Geometry: final body of the model. Coordinates: model frame, mm. A direction names the side the tool comes from. Give positions to 0.01 mm unless a question says otherwise; leave off trailing zeros. Loops run counter-clockwise (first coordinate to the right, second up) from the corner with the lowest first, then second, coordinate; pieces in that order, holes last. Notation, with made-up numbers: M 51.25,26 L 106.25,26 A11 cw 106.25,33 Z; hole C -19.75,53.5 d1. An arc over 180 degrees is marked long. Put each result on its own line as item: value.
```python
from build123d import *

# Parameters (mm, degrees)
ESBO_O1_W                = 30
ESBO_O1_H                = 30
RESSALTO_EXTRUS_O1_DEPTH = 28.5
ESBO_O2_R                = 1.6
CORTE_EXTRUS_O1_DEPTH    = 5
ESBO_O3_R                = 2.25
RESSALTO_EXTRUS_O2_DEPTH = 3
ESBO_O4_W                = 15.5
ESBO_O4_H                = 20
RESSALTO_EXTRUS_O3_DEPTH = 12
ESBO_O5_R                = 2.25
RESSALTO_EXTRUS_O4_DEPTH = 5
RESSALTO_EXTRUS_O4_TAPER = 22
ESBO_O6_W                = 30
ESBO_O6_H                = 30
ESBO_O6_W_2              = 29.5
ESBO_O6_H_2              = 29.5
ESBO_O6_R                = 14.4
CORTE_EXTRUS_O2_DEPTH    = 10.5
RESSALTO_EXTRUS_O5_DEPTH = 6
ESBO_O10_R               = 5
RESSALTO_EXTRUS_O6_DEPTH = 5.5


with BuildPart() as part:
    # Esboço1 → Ressalto-extrusão1 (new body)
    with BuildSketch(Plane.XY):
        Rectangle(ESBO_O1_W, ESBO_O1_H)
    extrude(amount=RESSALTO_EXTRUS_O1_DEPTH)

    # Esboço2 → Corte-extrusão1 (cut)
    with BuildSketch(Plane(origin=(0, 0, 0), x_dir=(-1, 0, 0), z_dir=(0, 0, -1))):
        with Locations((4.5, 5)):
            Circle(ESBO_O2_R)
        with Locations((-4.5, 5)):
            Circle(ESBO_O2_R)
        with Locations((0, -4.8)):
            Circle(ESBO_O2_R)
    extrude(amount=-CORTE_EXTRUS_O1_DEPTH, mode=Mode.SUBTRACT)

    # Esboço3 → Ressalto-extrusão2 (add)
    with BuildSketch(Plane.XZ.offset(15)):
        with Locations((-9, 5.5)):
            Circle(ESBO_O3_R)
        with Locations((9, 5.5)):
            Circle(ESBO_O3_R)
    extrude(amount=RESSALTO_EXTRUS_O2_DEPTH)

    # Esboço4 → Ressalto-extrusão3 (add)
    with BuildSketch(Plane.XZ.offset(18)):
        with Locations((-9, 12)):
            Rectangle(ESBO_O4_W, ESBO_O4_H)
        with Locations((9, 12)):
            Rectangle(ESBO_O4_W, ESBO_O4_H)
    extrude(amount=RESSALTO_EXTRUS_O3_DEPTH)

    # Esboço5 → Ressalto-extrusão4 (add)
    with BuildSketch(Plane.XZ.offset(30)):
        with Locations((9, 5.5)):
            Circle(ESBO_O5_R)
        with Locations((-9, 5.5)):
            Circle(ESBO_O5_R)
    extrude(amount=RESSALTO_EXTRUS_O4_DEPTH, taper=RESSALTO_EXTRUS_O4_TAPER)

    # Esboço6 → Corte-extrusão2 (cut)
    with BuildSketch(Plane.XY.offset(28.5)):
        Rectangle(ESBO_O6_W, ESBO_O6_H)
        Rectangle(ESBO_O6_W_2, ESBO_O6_H_2, mode=Mode.SUBTRACT)
        Circle(ESBO_O6_R)
        with BuildLine():
            ThreePointArc((-7.846216259, 2.549390204), (-8.188505751, 1.005422083), (-8.229903415, -0.575490908))
            Line((-8.229903415, -0.575490908), (-13.866140299, -0.969614985))
            ThreePointArc((-13.866140299, -0.969614985), (-12.157213929, -6.738853721), (-8.170215007, -11.245336222))
            Line((-8.170215007, -11.245336222), (-4.849228331, -6.674390204))
            ThreePointArc((-4.849228331, -6.674390204), (-3.486600659, -7.477039243), (-1.995855639, -8.004939742))
            Line((-1.995855639, -8.004939742), (-3.362714349, -13.487110595))
            ThreePointArc((-3.362714349, -13.487110595), (2.652245036, -13.64461785), (8.170215007, -11.245336222))
            Line((8.170215007, -11.245336222), (4.849228331, -6.674390204))
            ThreePointArc((4.849228331, -6.674390204), (6.033668038, -5.626486471), (6.996396793, -4.37183393))
            Line((6.996396793, -4.37183393), (11.787868537, -7.365877773))
            ThreePointArc((11.787868537, -7.365877773), (13.796391508, -1.693983873), (13.219685577, 4.295336222))
            Line((13.219685577, 4.295336222), (7.846216259, 2.549390204))
            ThreePointArc((7.846216259, 2.549390204), (7.215612584, 3.999679367), (6.319866656, 5.30299778))
            Line((6.319866656, 5.30299778), (10.648017759, 8.934747775))
            ThreePointArc((10.648017759, 8.934747775), (5.874393838, 12.59767824), (0, 13.9))
            Line((0, 13.9), (0, 8.25))
            ThreePointArc((0, 8.25), (-1.574174212, 8.098424263), (-3.090504396, 7.6492668))
            Line((-3.090504396, 7.6492668), (-5.207031648, 12.887855578))
            ThreePointArc((-5.207031648, 12.887855578), (-10.165816453, 9.479777205), (-13.219685577, 4.295336222))
            Line((-13.219685577, 4.295336222), (-7.846216259, 2.549390204))
        make_face(mode=Mode.SUBTRACT)
    extrude(amount=-CORTE_EXTRUS_O2_DEPTH, mode=Mode.SUBTRACT)

    # Esboço9 → Ressalto-extrusão5 (add)
    with BuildSketch(Plane(origin=(0, 15, 0), x_dir=(1, 0, 0), z_dir=(0, 1, 0))):
        Polygon((14.773502692, -5.5), (11.886751346, -0.5), (6.113248654, -0.5), (3.226497308, -5.5), (6.113248654, -10.5), (11.886751346, -10.5), align=None)
        Polygon((-3.226497308, -5.5), (-6.113248654, -0.5), (-11.886751346, -0.5), (-14.773502692, -5.5), (-11.886751346, -10.5), (-6.113248654, -10.5), align=None)
    extrude(amount=RESSALTO_EXTRUS_O5_DEPTH)

    # Esboço10 → Ressalto-extrusão6 (add)
    with BuildSketch(Plane(origin=(0, 21, 0), x_dir=(1, 0, 0), z_dir=(0, 1, 0))):
        with Locations((-9, -5.5)):
            Circle(ESBO_O10_R)
        with Locations((9, -5.5)):
            Circle(ESBO_O10_R)
    extrude(amount=RESSALTO_EXTRUS_O6_DEPTH)


solid = part.part
```
Item 1: Line query: probe 1 along Y at (x, z) = (0, 3.1); probe 2 along Y at (x, z) = (-2, 6.25); probe 3 along X at (y, z) = (12, 21.5). Output: solid intervals per line, ascending. Write a range as [from, to].
Output values:
probe 1: [-15, -6.4], [-3.2, 15]
probe 2: [-30, -18], [-15, 15]
probe 3: [-14.75, -7.96], [-7.01, -4.85], [0, 7.01], [7.96, 14.75]
Item 2: Section C-C on z = 14.25. Output: boundary loops of the cut face in (x, y), then the cut area to 3 significant figures.
Output values:
outline: M -16.75,-30 L -1.25,-30 L -1.25,-18 L -16.75,-18 Z; M -15,-15 L 15,-15 L 15,15 L -15,15 Z; M 1.25,-30 L 16.75,-30 L 16.75,-18 L 1.25,-18 Z
area: 1,270 mm²
Item 3: Mould query, pull axis Y, two halves, no side actions, for faces 5 (the flat face through (13.31, 17.958, 8.035)), 6 (the flat face through (0, -5, 5)), 7 (the flat face through (6, 21, 10)). Classes: pulls with the +Y half, pulls with the -Y half, needs draft (parallel to the pull), parting line crosses it, or undercut.
Output values:
face 5: needs draft
face 6: undercut
face 7: pulls with the +Y half
Item 4: Section B-B on z = 24.5. Output: boundary loops of the cut face in (x, y), then the cut area to 3 significant figures.
Output values:
outline: M -14.75,-14.75 L 14.75,-14.75 L 14.75,14.75 L -14.75,14.75 Z; M -13.87,-0.97 A13.9 ccw -8.17,-11.25 L -4.85,-6.67 A8.25 ccw -2,-8 L -3.36,-13.49 A13.9 ccw 8.17,-11.25 L 4.85,-6.67 A8.25 ccw 7,-4.37 L 11.79,-7.37 A13.9 ccw 13.22,4.3 L 7.85,2.55 A8.25 ccw 6.32,5.3 L 10.65,8.93 A13.9 ccw 0,13.9 L 0,8.25 A8.25 ccw -3.09,7.65 L -5.21,12.89 A13.9 ccw -13.22,4.3 L -7.85,2.55 A8.25 ccw -8.23,-0.58 Z; hole C 0,0 d28.8
area: 706 mm²
Item 5: Set-up query: faces 1 (the cylindrical face through (-4.15, 3.44, 2.46)), 2 (the flat face through (0, -14.75, 23)), 3 (the flat face through (14.2, 21, 5.5)), 4 (the flat face through (-4.134, 10.232, 23.324)). Return all of +Z, -Z, +X, -X, +Y, -Y with unobstructed straight access to the full face (end or side cutting, diameter ignored); none if empty.
Output values:
face 1: -Z
face 2: +Z, +X, -X
face 3: +X, +Y
face 4: +Z
Item 6: Section A-A on z = 21. Count the separate pieces of the cut face and the enclosed holes in it, then the cut area to 3 significant figures.
Output values:
separate pieces: 4
enclosed holes: 1
area: 1,080 mm²
Item 7: Pin query (flat end, axial travel): pin 1 Ø1 at (x, z) = (12, 12.5) entering from -Y; pin 2 Ø10 at (y, z) = (3.5, 12.5) entering from -X; pin 3 Ø3 at (x, y) = (-4.5, 5) entering from -Z. Return the tip coordinate at first contact, or that it passes through.
Output values:
pin 1: y = -30
pin 2: x = -15
pin 3: z = 5
